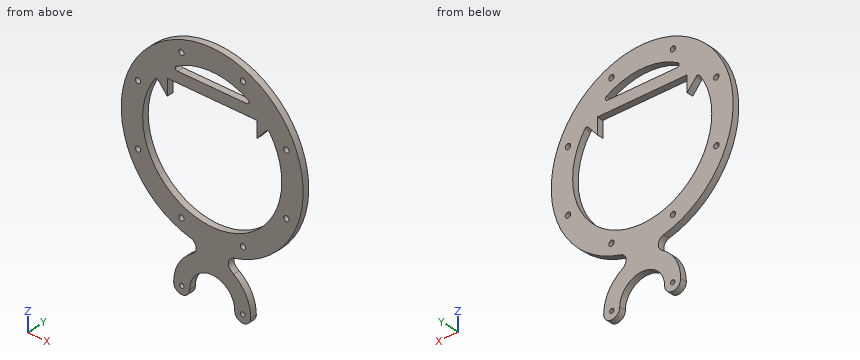
Autodesk Inventor part; units mm, degrees
ref_plane "YZ Plane" through (0, 0, 0) normal (1, 0, 0) x (0, 1, 0)
ref_plane "XZ Plane" through (0, 0, 0) normal (0, 1, 0) x (-1, 0, 0)
ref_plane "XY Plane" through (0, 0, 0) normal (0, 0, 1) x (1, 0, 0)
sketch "Sketch1" plane through (0, 0, 0) normal (0, 1, 0) x (-1, 0, 0)
  arc A0 (20, -82.6136) -> (-20, -82.6136) centre (0, 0) ccw
  line L0 (0, 0) -> (0, -85)
  line L1 (0, 0) -> (32.5281, -78.5298)
  circle A1 centre (0, 0) radius 75 construction
  circle A2 centre (28.7013, -69.291) radius 2.5
  line L2 (41, -41) -> (-41, -41) construction
  line L3 (-41, -41) -> (-41, 41) construction
  line L4 (-41, 41) -> (41, 41) construction
  line L5 (41, 41) -> (41, -41) construction
  line L6 (0, 0) -> (-85, 0)
  circle A3 centre (69.291, -28.7013) radius 2.5
  circle A4 centre (69.291, 28.7013) radius 2.5
  circle A5 centre (28.7013, 69.291) radius 2.5
  circle A6 centre (-28.7013, 69.291) radius 2.5
  circle A7 centre (-69.291, 28.7013) radius 2.5
  circle A8 centre (-69.291, -28.7013) radius 2.5
  circle A9 centre (-28.7013, -69.291) radius 2.5
  line L7 (42, 27) -> (42, 42)
  line L8 (42, 42) -> (-42, 42)
  line L9 (-42, 42) -> (-42, 27)
  line L10 (42, 27) -> (52.0326, 38.9564)
  line L11 (-39, 52) -> (39, 52)
  line L12 (-42, 27) -> (-52.0326, 38.9564)
  arc A10 (-52.0326, 38.9564) -> (52.0326, 38.9564) centre (0, 0) ccw
  arc A11 (39, 52) -> (-39, 52) centre (0, 0) ccw
  arc A12 (21, -126) -> (-21, -126) centre (0, -126) ccw
  line L13 (0, -105) -> (0, -85) construction
  arc A13 (-20, -82.6136) -> (20, -82.6136) centre (0, 0) ccw construction
  line L14 (0, -126) -> (36, -126) construction
  arc A14 (27.5132, -133.4348) -> (-27.5132, -133.4348) centre (0, -126) ccw
  circle A15 centre (28.5, -126) radius 2
  circle A16 centre (-28.5, -126) radius 2
  arc A17 (-20, -96.0667) -> (-36, -126) centre (0, -126) ccw
  arc A18 (36, -126) -> (20, -96.0667) centre (0, -126) ccw
  arc A19 (21, -126) -> (36, -126) centre (28.5, -126) ccw
  line L15 (0, -126) -> (-36, -126) construction
  arc A20 (-36, -126) -> (-21, -126) centre (-28.5, -126) ccw
  line L16 (-20, -89.3401) -> (-15, -89.3401) construction
  spline S0 degree 4 poles (-20, -82.6136) (-15.4558, -83.7137) (-12.0866, -90.2039) (-16.4143, -93.671) (-20, -96.0667) knots 0 0 0 0 0 1 1 1 1 1
  spline S1 degree 4 poles (20, -82.6136) (15.4558, -83.7137) (12.0866, -90.2039) (16.4143, -93.671) (20, -96.0667) knots 0 0 0 0 0 1 1 1 1 1
  line L17 (20, -89.3401) -> (15, -89.3401) construction
  line L18 (20, -96.0667) -> (20, -82.6136) construction
  line L19 (-20, -96.0667) -> (-20, -82.6136) construction
  point P0 (0, -41)
  point P1 (-41, 0)
  point P2 (0, 52)
  point P3 (17.5, -89.3401)
  dimension "d4" = 150
  dimension "d0" = 170
  dimension "d3" = 22.5
  dimension "d6" = 82
  dimension "d10" = 360
  dimension "d12" = 5
  dimension "d13" = 1
  dimension "d14" = 1
  dimension "d15" = 1
  dimension "d16" = 15
  dimension "d17" = 40
  dimension "d18" = 10
  dimension "d19" = 40
  dimension "d20" = 20
  dimension "d21" = 42
  dimension "d25" = 20
  dimension "d28" = 57
  dimension "d32" = 360
  dimension "d34" = 4
  dimension "d37" = 15
  dimension "d41" = 5
  dimension "d42" = 6.7266
  dimension "d43" = 6.7266
  dimension "d44" = 30
extrude "Extrusion1" add sketch "Sketch1" along normal blind 6 contours S1 A18 A19 A14 A15 A16 A20 A17 S0 A0 L6 A10 L1 A2 | L1 A2 A10 L10 L7 L8 L9 L12 L6 A0 | A19 A12 A20 A14 A16 A15
sketch "Sketch2" plane through (0, 6, 0) normal (0, 1, 0) x (1, 0, 0)
  point P0 (0, 0)
fillet "Fillet1" radius 2 4 edges at (-39, 3, 52) (39, 3, 52) (-52.0326, 3, 38.9564) (52.0326, 3, 38.9564)
equation "\"d14\" = d13"
equation "\"d15\" = d13"
equation "\"d19\" = d17"
properties part number "SparRing Curved" material "Plywood, Finish"
Design review of the part built by this model. Coordinates are the model's own, in mm. Coordinates: 2 decimals unless noted, no trailing zeros. Write each loop counter-clockwise with the first axis right and the second up, starting at its lowest first coordinate (ties: lowest second). Pieces come first, ordered by that corner, then holes. Notation, with made-up numbers: (-15, 11.5) - (16, 11.5) arc R32 cw to (16, 44.5) - close; hole circle Ø5 at (2, 28). An arc over 180 degrees is marked (long way). Use one line per item in the form item = value.
Q1. Consider section A-A (x = 0). Write out the cut boundary in (y, z), plus the area to 3 significant figures.
Taken from the geometry:
outline = (0, -105) - (6, -105) - (6, -65) - (0, -65) - close; (0, 42) - (6, 42) - (6, 52) - (0, 52) - close; (0, 65) - (6, 65) - (6, 85) - (0, 85) - close
area = 420 mm^2
Q2. Consider section D-D (y = 2.5). Count the separate pieces of the cut face and the enclosed holes in it, plus the area to 3 significant figures.
Taken from the geometry:
separate_pieces = 1
enclosed_holes = 12
area = 12,100 mm^2
Q3. Consider section B-B (z = -14.5). Write out the cut boundary in (x, y).
Taken from the geometry:
outline = (-83.75, 0) - (-63.36, 0) - (-63.36, 6) - (-83.75, 6) - close; (63.36, 0) - (83.75, 0) - (83.75, 6) - (63.36, 6) - close
Q4. Insertion check: pin 1 Ø3.5 at (x, z) = (-28.5, -126) entering from +Y; pin 2 Ø3 at (x, y) = (-10.5, 3.5) entering from +Z; pin 3 Ø1 at (y, z) = (3.5, 9.5) entering from -X; pin 4 Ø1 at (x, y) = (-52, 0.5) entering from +Z. Each pin has a flat end and moves straight along its axis. Give the tip position at first contact, or say it passes through.
Taken from the geometry:
pin_1 = through
pin_2 = 84.52
pin_3 = -84.52
pin_4 = 67.62
Q5. For probe 1 along Z at (x, y) = (0.5, 1.5); probe 2 along Z at (x, y) = (2.5, 2.5); probe 3 along Z at (x, y) = (40.5, 2.5), list the stretches that pass through material, from the lowest coordinate up.
Taken from the geometry:
probe_1 = -105.01 to -65, 42 to 52, 65 to 85
probe_2 = -105.15 to -64.95, 42 to 52, 64.95 to 84.96
probe_3 = -74.73 to -50.84, 42 to 74.73
Q6. Consider section C-C (x = -57). Write out the cut boundary in (y, z).
Taken from the geometry:
outline = (0, -63.06) - (6, -63.06) - (6, -31.24) - (0, -31.24) - close; (0, 31.24) - (6, 31.24) - (6, 63.06) - (0, 63.06) - close
